```python
from build123d import *

# Parameters (mm, degrees)
SKETCH1_W           = 30
SKETCH1_H           = 5
SKETCH1_W_2         = 20
BOSS_EXTRUDE1_DEPTH = 5


with BuildPart() as part:
    # Sketch1 → Boss-Extrude1 (new body)
    with BuildSketch(Plane.XY):
        Polygon((84.753464523, -219.784412909), (-375.246535477, -219.784412909), (-375.246535477, -194.784412909), (-370.246535477, -194.784412909), (-370.246535477, -174.784412909), (-375.246535477, -174.784412909), (-375.246535477, -149.784412909), (-370.246535477, -149.784412909), (-370.246535477, -129.784412909), (-375.246535477, -129.784412909), (-375.246535477, -104.784412909), (-370.246535477, -104.784412909), (-370.246535477, -84.784412909), (-375.246535477, -84.784412909), (-375.246535477, -54.784412909), (-370.246535477, -54.784412909), (-370.246535477, -34.784412909), (-375.246535477, -34.784412909), (-375.246535477, -9.784412909), (-370.246535477, -9.784412909), (-370.246535477, 10.215587091), (-375.246535477, 10.215587091), (-375.246535477, 35.215587091), (-370.246535477, 35.215587091), (-370.246535477, 55.215587091), (-375.246535477, 55.215587091), (-375.246535477, 80.215587091), (84.753464523, 80.215587091), (84.753464523, 55.215587091), (79.753464523, 55.215587091), (79.753464523, 35.215587091), (84.753464523, 35.215587091), (84.753464523, 10.215587091), (79.753464523, 10.215587091), (79.753464523, -9.784412909), (84.753464523, -9.784412909), (84.753464523, -34.784412909), (79.753464523, -34.784412909), (79.753464523, -54.784412909), (84.753464523, -54.784412909), (84.753464523, -84.784412909), (79.753464523, -84.784412909), (79.753464523, -104.784412909), (84.753464523, -104.784412909), (84.753464523, -129.784412909), (79.753464523, -129.784412909), (79.753464523, -149.784412909), (84.753464523, -149.784412909), (84.753464523, -174.784412909), (79.753464523, -174.784412909), (79.753464523, -194.784412909), (84.753464523, -194.784412909), align=None)
        with Locations((-70.246535477, -207.284412909)):
            Rectangle(SKETCH1_W, SKETCH1_H, mode=Mode.SUBTRACT)
        with Locations((-120.246535477, -207.284412909)):
            Rectangle(SKETCH1_W, SKETCH1_H, mode=Mode.SUBTRACT)
        with Locations((-20.246535477, -207.284412909)):
            Rectangle(SKETCH1_W, SKETCH1_H, mode=Mode.SUBTRACT)
        with Locations((29.753464523, -207.284412909)):
            Rectangle(SKETCH1_W, SKETCH1_H, mode=Mode.SUBTRACT)
        with Locations((-320.246535477, -207.284412909)):
            Rectangle(SKETCH1_W, SKETCH1_H, mode=Mode.SUBTRACT)
        with Locations((-270.246535477, -207.284412909)):
            Rectangle(SKETCH1_W, SKETCH1_H, mode=Mode.SUBTRACT)
        with Locations((-220.246535477, -207.284412909)):
            Rectangle(SKETCH1_W, SKETCH1_H, mode=Mode.SUBTRACT)
        with Locations((-170.246535477, -207.284412909)):
            Rectangle(SKETCH1_W, SKETCH1_H, mode=Mode.SUBTRACT)
        with Locations((-220.246535477, 67.715587091)):
            Rectangle(SKETCH1_W, SKETCH1_H, mode=Mode.SUBTRACT)
        with Locations((-170.246535477, 67.715587091)):
            Rectangle(SKETCH1_W, SKETCH1_H, mode=Mode.SUBTRACT)
        with Locations((-270.246535477, 67.715587091)):
            Rectangle(SKETCH1_W, SKETCH1_H, mode=Mode.SUBTRACT)
        with Locations((-320.246535477, 67.715587091)):
            Rectangle(SKETCH1_W, SKETCH1_H, mode=Mode.SUBTRACT)
        with Locations((29.753464523, 67.715587091)):
            Rectangle(SKETCH1_W, SKETCH1_H, mode=Mode.SUBTRACT)
        with Locations((-20.246535477, 67.715587091)):
            Rectangle(SKETCH1_W, SKETCH1_H, mode=Mode.SUBTRACT)
        with Locations((-70.246535477, 67.715587091)):
            Rectangle(SKETCH1_W, SKETCH1_H, mode=Mode.SUBTRACT)
        with Locations((-120.246535477, 67.715587091)):
            Rectangle(SKETCH1_W, SKETCH1_H, mode=Mode.SUBTRACT)
        with Locations((-185.246535477, -69.784412909)):
            Rectangle(SKETCH1_W_2, SKETCH1_H, mode=Mode.SUBTRACT)
        with Locations((-145.246535477, -69.784412909)):
            Rectangle(SKETCH1_W_2, SKETCH1_H, mode=Mode.SUBTRACT)
        with Locations((-225.246535477, -69.784412909)):
            Rectangle(SKETCH1_W_2, SKETCH1_H, mode=Mode.SUBTRACT)
        with Locations((-265.246535477, -69.784412909)):
            Rectangle(SKETCH1_W_2, SKETCH1_H, mode=Mode.SUBTRACT)
        with Locations((-305.246535477, -69.784412909)):
            Rectangle(SKETCH1_W_2, SKETCH1_H, mode=Mode.SUBTRACT)
        with Locations((-345.246535477, -69.784412909)):
            Rectangle(SKETCH1_W_2, SKETCH1_H, mode=Mode.SUBTRACT)
        with Locations((54.753464523, -69.784412909)):
            Rectangle(SKETCH1_W_2, SKETCH1_H, mode=Mode.SUBTRACT)
        with Locations((14.753464523, -69.784412909)):
            Rectangle(SKETCH1_W_2, SKETCH1_H, mode=Mode.SUBTRACT)
        with Locations((-25.246535477, -69.784412909)):
            Rectangle(SKETCH1_W_2, SKETCH1_H, mode=Mode.SUBTRACT)
        with Locations((-65.246535477, -69.784412909)):
            Rectangle(SKETCH1_W_2, SKETCH1_H, mode=Mode.SUBTRACT)
        with Locations((-105.246535477, -69.784412909)):
            Rectangle(SKETCH1_W_2, SKETCH1_H, mode=Mode.SUBTRACT)
    extrude(amount=BOSS_EXTRUDE1_DEPTH)


solid = part.part
```
Geometry: final body of the model. Coordinates: model frame, mm. Give positions to 0.01 mm unless a question says otherwise; leave off trailing zeros. Order: outer loops, then holes, each group sorted by start corner. A loop starts at its lowest first (then second) coordinate and runs counter-clockwise, first axis right, second up. Notation, with made-up numbers: M 85,-23.75 L 132,-23.75 A21 ccw 132,-7.75 Z; hole C 21,-25 d2. An arc over 180 degrees is marked long. Answer as CSV lines item,"result". Start each with the question number.
1) Cut plane C-C (y = -137.5). Output: boundary loops of the cut face in (x, z), then the cut area to 3 significant figures.
2) First-contact query: P1, Ø2.5, axis at y = -184, z = 1.5, coming from the -X side. Flat tip, straight axial feed; report the tip coordinate or a pass-through.
3) Line query: line 1 (Y direction, x = -265.5, z = 4.6); line 2 (Y direction, x = -13, z = 3.45); line 3 (Y direction, x = -301, z = 2.4). Output: solid intervals per line, ascending. Write a range as from..to.
4) Cut plane B-B (z = 1.35). State how many separate pieces and enclosed holes the cut face has, then the cut area to 3 significant figures.
5) Cut plane A-A (x = -344). Output: boundary loops of the cut face in (y, z), then the cut area to 4 significant figures.
Findings below:
1,outline,"M -370.25,0 L 79.75,0 L 79.75,5 L -370.25,5 Z"
1,area,"2,250 mm²"
2,P1,"stops at x = -370.25"
3,line 1,"y = -219.78..-209.78, -204.78..-72.28, -67.28..65.22, 70.22..80.22"
3,line 2,"y = -219.78..-209.78, -204.78..65.22, 70.22..80.22"
3,line 3,"y = -219.78..-72.28, -67.28..80.22"
4,separate pieces,"1"
4,enclosed holes,"27"
4,area,"133,000 mm²"
5,outline,"M -219.78,0 L -72.28,0 L -72.28,5 L -219.78,5 Z; M -67.28,0 L 80.22,0 L 80.22,5 L -67.28,5 Z"
5,area,"1,475 mm²"
